CAD build for the part. Positions are in the model's coordinates, mm. Face numbers are marked on the shaded views. Coordinates: 2 decimals unless noted, no trailing zeros. Order: outer loops, then holes, each group sorted by start corner. A loop starts at its lowest first (then second) coordinate and runs counter-clockwise, first axis right, second up. Notation, with made-up numbers: M 68,66 L 94,66 A25 ccw 94,96 Z; hole C 37,18 d8. An arc over 180 degrees is marked long. Write item = value, one per line.
from build123d import *

# Parameters (mm, degrees)
SKETCH1_W           = 142.5
SKETCH1_H           = 94
BOSS_EXTRUDE1_DEPTH = 15
SKETCH2_W           = 126.5
SKETCH2_H           = 78
CUT_EXTRUDE2_DEPTH  = 3
CHAMFER1_SIZE       = 2
SKETCH6_R           = 2.5
CUT_EXTRUDE7_DEPTH  = 10
SKETCH7_R           = 5
CUT_EXTRUDE8_DEPTH  = 5
CHAMFER2_SIZE       = 3
SKETCH8_R           = 10
CUT_EXTRUDE9_DEPTH  = 15
CUT_EXTRUDE10_DEPTH = 172.368754445


# Some blends are built 0.0001 mm under size
with BuildPart() as part:
    # Sketch1 → Boss-Extrude1 (new body)
    with BuildSketch(Plane(origin=(0, 0, 0), x_dir=(1, 0, 0), z_dir=(0, 1, 0))):
        with Locations((71.25, 47)):
            Rectangle(SKETCH1_W, SKETCH1_H)
    extrude(amount=BOSS_EXTRUDE1_DEPTH)

    # Sketch2 → Cut-Extrude2 (cut)
    with BuildSketch(Plane(origin=(0, 15, 0), x_dir=(1, 0, 0), z_dir=(0, 1, 0))):
        Polygon((134.5, 92), (8, 92), (8, 94), (2, 94), (2, 0), (8, 0), (8, 2), (134.5, 2), (134.5, 0), (140.5, 0), (140.5, 94), (134.5, 94), align=None)
        with Locations((71.25, 47)):
            Rectangle(SKETCH2_W, SKETCH2_H, mode=Mode.SUBTRACT)
    extrude(amount=-CUT_EXTRUDE2_DEPTH, mode=Mode.SUBTRACT)

    # Chamfer1
    chamfer1_edges = [part.edges().sort_by_distance(p)[0] for p in [
        (0, 7.5, 0),
        (0, 7.5, -94),
        (142.5, 7.5, -94),
        (142.5, 7.5, 0),
    ]]
    chamfer(chamfer1_edges, length=CHAMFER1_SIZE - 0.0001)  # a hair under: the kernel refuses the full size

    # Sketch6 → Cut-Extrude7 (cut)
    with BuildSketch(Plane(origin=(0, 15, 0), x_dir=(1, 0, 0), z_dir=(0, 1, 0))):
        with Locations(Location((124.5, 75, 0), (0, 0, 270))):
            Circle(SKETCH6_R)
        with Locations(Location((18, 75, 0), (0, 0, 270))):
            Circle(SKETCH6_R)
        with Locations(Location((18, 19, 0), (0, 0, 270))):
            Circle(SKETCH6_R)
        with Locations(Location((124.5, 19, 0), (0, 0, 270))):
            Circle(SKETCH6_R)
    extrude(amount=-CUT_EXTRUDE7_DEPTH, mode=Mode.SUBTRACT)

    # Sketch7 → Cut-Extrude8 (cut)
    with BuildSketch(Plane.XZ):
        with Locations(Location((18, -19, 0), (0, 0, 270))):
            Circle(SKETCH7_R)
        with Locations(Location((124.5, -19, 0), (0, 0, 270))):
            Circle(SKETCH7_R)
        with Locations(Location((18, -75, 0), (0, 0, 270))):
            Circle(SKETCH7_R)
        with Locations(Location((124.5, -75, 0), (0, 0, 270))):
            Circle(SKETCH7_R)
    extrude(amount=-CUT_EXTRUDE8_DEPTH, mode=Mode.SUBTRACT)

    # Chamfer2
    # the kernel refuses this chamfer: 3 mm, written as the material it takes off along each edge
    with BuildSketch(Plane(origin=(142.5, 0, 5.715148964), x_dir=(-0.9996219169112968, -0.027495876610586487, 0), z_dir=(0, 0, -1)), Plane(origin=(0, 0, -99.715148964), x_dir=(0.9996219169112968, -0.027495876610586372, 0), z_dir=(0, 0, 1))) as chamfer2_piece_1:
        Polygon((CHAMFER2_SIZE * 0.999621916911, CHAMFER2_SIZE * 0.0274958766106), (-CHAMFER2_SIZE * 0.0274958766106, CHAMFER2_SIZE * 0.999621916911), (0, 0), align=None)
    extrude(amount=105.430297928, mode=Mode.SUBTRACT)
    with BuildSketch(Plane(origin=(-5.715148964, 0, 0), x_dir=(0, 0.9996219169112968, 0.027495876610586372), z_dir=(1, 0, 0))) as chamfer2_piece_2:
        Polygon((CHAMFER2_SIZE * 0.999621916911, -CHAMFER2_SIZE * 0.0274958766106), (-CHAMFER2_SIZE * 0.0274958766106, -CHAMFER2_SIZE * 0.999621916911), (0, 0), align=None)
    extrude(amount=153.930297928, mode=Mode.SUBTRACT)
    with BuildSketch(Plane(origin=(148.215148964, 0, -94), x_dir=(0, -0.02749587661058636, 0.9996219169112968), z_dir=(-1, 0, 0))) as chamfer2_piece_3:
        Polygon((CHAMFER2_SIZE * 0.999621916911, CHAMFER2_SIZE * 0.0274958766106), (-CHAMFER2_SIZE * 0.0274958766106, CHAMFER2_SIZE * 0.999621916911), (0, 0), align=None)
    extrude(amount=153.930297928, mode=Mode.SUBTRACT)

    # Sketch8 → Cut-Extrude9 (cut)
    with BuildSketch(Plane(origin=(0, 15, 0), x_dir=(1, 0, 0), z_dir=(0, 1, 0))):
        with Locations(Location((71.25, 47, 0), (0, 0, 270))):
            Circle(SKETCH8_R)
    extrude(amount=-CUT_EXTRUDE9_DEPTH, mode=Mode.SUBTRACT)

    # Sketch9 → Cut-Extrude10 (cut, through all)
    with BuildSketch(Plane(origin=(0, 15, 0), x_dir=(1, 0, 0), z_dir=(0, 1, 0))):
        with BuildLine():
            Line((54.75, 60.75), (54.75, 63.5))
            Line((54.75, 63.5), (57.5, 63.5))
            ThreePointArc((57.5, 63.5), (52.805456352, 65.444543648), (54.75, 60.75))
        make_face()
        with BuildLine():
            Line((57.5, 63.5), (54.75, 63.5))
            Line((54.75, 63.5), (54.75, 60.75))
            ThreePointArc((54.75, 60.75), (56.694543648, 61.555456352), (57.5, 63.5))
        make_face()
        with BuildLine():
            ThreePointArc((57.5, 30.5), (56.694543648, 32.444543648), (54.75, 33.25))
            Line((54.75, 33.25), (54.75, 30.5))
            Line((54.75, 30.5), (57.5, 30.5))
        make_face()
        with BuildLine():
            Line((54.75, 30.5), (54.75, 33.25))
            ThreePointArc((54.75, 33.25), (52.805456352, 28.555456352), (57.5, 30.5))
            Line((57.5, 30.5), (54.75, 30.5))
        make_face()
        with BuildLine():
            ThreePointArc((90.5, 30.5), (89.694543648, 32.444543648), (87.75, 33.25))
            Line((87.75, 33.25), (87.75, 30.5))
            Line((87.75, 30.5), (85, 30.5))
            ThreePointArc((85, 30.5), (87.75, 27.75), (90.5, 30.5))
        make_face()
        with BuildLine():
            Line((87.75, 30.5), (87.75, 33.25))
            ThreePointArc((87.75, 33.25), (85.805456352, 32.444543648), (85, 30.5))
            Line((85, 30.5), (87.75, 30.5))
        make_face()
        with BuildLine():
            ThreePointArc((90.5, 63.5), (87.75, 66.25), (85, 63.5))
            Line((85, 63.5), (87.75, 63.5))
            Line((87.75, 63.5), (87.75, 60.75))
            ThreePointArc((87.75, 60.75), (89.694543648, 61.555456352), (90.5, 63.5))
        make_face()
        with BuildLine():
            Line((87.75, 63.5), (85, 63.5))
            ThreePointArc((85, 63.5), (85.805456352, 61.555456352), (87.75, 60.75))
            Line((87.75, 60.75), (87.75, 63.5))
        make_face()
    extrude(amount=-CUT_EXTRUDE10_DEPTH, mode=Mode.SUBTRACT)


solid = part.part
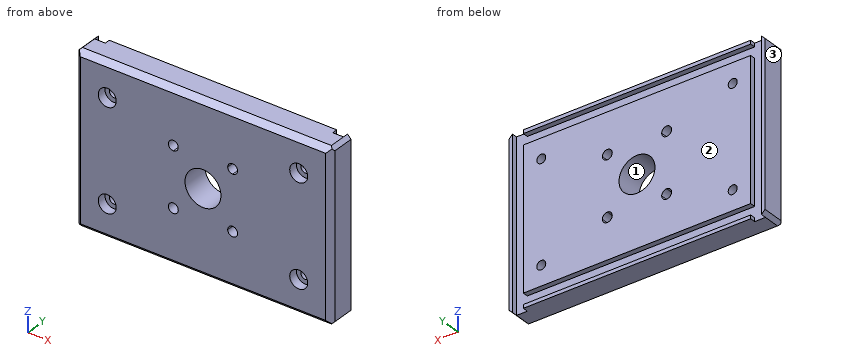
(1) Slice it at A-A, the plane z = -75. State how many separate pieces and enclosed holes the cut face has, then the cut area to 3 significant figures.
Evaluation:
separate_pieces = 3
enclosed_holes = 0
area = 1,890 mm²
(2) Pull direction X, two halves, no side cores. Call the marked faces 1, 2 and 3: +X half, -X half, draft (parallel to the pull), parting line (faces both ways), or undercut.
Evaluation:
face_1 = undercut
face_2 = draft
face_3 = -X half
(3) Pin check, flat tips, straight feed: pin 1 Ø8 at (x, z) = (19.5, -73) entering from -Y; pin 2 Ø1 at (y, z) = (13.5, -1) entering from +X; pin 3 Ø8 at (x, z) = (124.5, -75) entering from -Y; pin 4 Ø0.6 at (y, z) = (13, -0.5) entering from -X. Stop position of each tip, or through.
Evaluation:
pin_1 = 0
pin_2 = 142
pin_3 = 5
pin_4 = 1.2
(4) Wall check: line 1 (X direction, y = 6.75, z = -30.5); line 2 (Z direction, x = 54.75, y = 11); line 3 (X direction, y = 3.15, z = -19). Give the ranges that are in metal, low to high. Write a range as from..to.
Evaluation:
line_1 = 0..52, 57.5..85, 90.5..142.5
line_2 = -94..-66.25, -60.75..-33.25, -27.75..0
line_3 = 0..13, 23..119.5, 129.5..142.5
(5) Slice it at B-B, the plane x = 71.25. Write the cut outline in (y, z).
Evaluation:
outline = M 0,-91 L 3,-94 L 15,-94 L 15,-92 L 12,-92 L 12,-86 L 15,-86 L 15,-57 L 0,-57 Z; M 0,-37 L 15,-37 L 15,-8 L 12,-8 L 12,-2 L 15,-2 L 15,0 L 3,0 L 0,-3 Z
